The drawing under review shows one solid part. Ordinate dimensions are in mm from its lowest x, y, z. Give positions to 0.01 mm unless a question says otherwise; leave off trailing zeros. Order: outer loops, then holes, each group sorted by start corner. A loop starts at its lowest first (then second) coordinate and runs counter-clockwise, first axis right, second up. Notation, with made-up numbers: (-26.75, 82.25) -> (29.25, 82.25) arc R25 cw to (29.25, 109.25) -> close; hole circle Ø10 at (58, -32). An arc over 180 degrees is marked (long way). One line per item, written item: value.
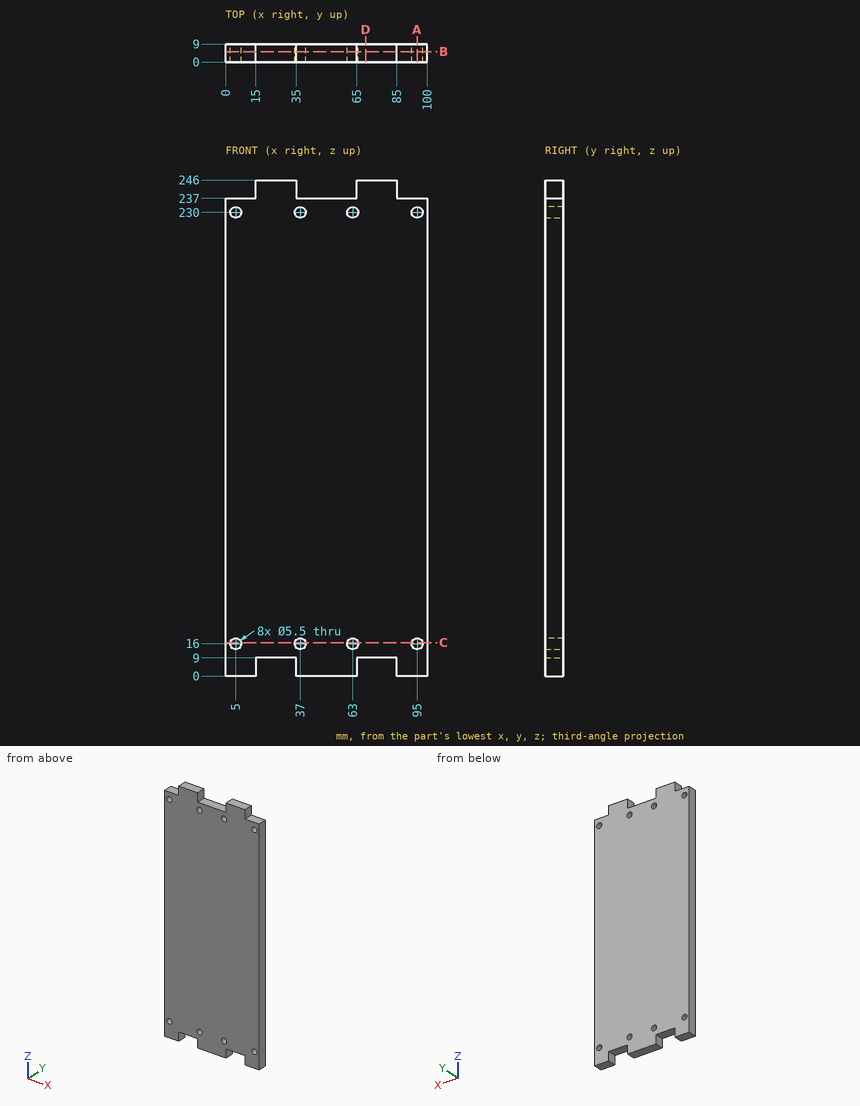
Item 1: Clearance check with flat-ended pins moving along their axes: P1, Ø5, axis at x = 63, z = 230, coming from the +Y side; P2, Ø5, axis at x = 44, y = 7, coming from the +Z side; P3, Ø1, axis at x = 80, y = 1.5, coming from the -Z side; P4, Ø4.5, axis at y = 6, z = 239.5, coming from the +X side. State where each tip first meets the part, or that it passes through.
Returned:
P1: through
P2: z = 237
P3: z = 9
P4: x = 85
Item 2: Add section A-A on x = 95. Give the boundary of the cut face in (y, z).
Returned:
outline: (0, 0) -> (9, 0) -> (9, 13.25) -> (0, 13.25) -> close; (0, 18.75) -> (9, 18.75) -> (9, 227.25) -> (0, 227.25) -> close; (0, 232.75) -> (9, 232.75) -> (9, 237) -> (0, 237) -> close
Item 3: Add section C-C on z = 16.5. Give the boundary of the cut face in (x, y).
Returned:
outline: (0, 0) -> (2.3, 0) -> (2.3, 9) -> (0, 9) -> close; (7.7, 0) -> (34.3, 0) -> (34.3, 9) -> (7.7, 9) -> close; (39.7, 0) -> (60.3, 0) -> (60.3, 9) -> (39.7, 9) -> close; (65.7, 0) -> (92.3, 0) -> (92.3, 9) -> (65.7, 9) -> close; (97.7, 0) -> (100, 0) -> (100, 9) -> (97.7, 9) -> close
Item 4: Add section D-D on x = 69.5. Give the boundary of the cut face in (y, z).
Returned:
outline: (0, 9) -> (9, 9) -> (9, 246) -> (0, 246) -> close
Item 5: To check wall thickness, follow line 1 along X through (y, z) = (6.25, 230); line 2 along Z through (x, y) = (18.5, 6.75); line 3 along Z through (x, y) = (48.5, 4.5). State the ranges of each line that lie inside material, in increasing order. Write a range as from..to.
Returned:
line 1: 0..2.25, 7.75..34.25, 39.75..60.25, 65.75..92.25, 97.75..100
line 2: 9..246
line 3: 0..237
Item 6: Add section B-B on y = 5.25. Count the separate pieces of the cut face and the enclosed holes in it, plus the area to 3 significant figures.
Returned:
separate pieces: 1
enclosed holes: 8
area: 23,500 mm²
